Read the model definition and answer for the solid it produces. Units are mm, in the model's axes. A direction names the side the tool comes from. Coordinates: 2 decimals unless noted, no trailing zeros. Loops run counter-clockwise (first coordinate to the right, second up) from the corner with the lowest first, then second, coordinate; pieces in that order, holes last. Notation, with made-up numbers: (11, 5.25) - (30, 5.25) arc R25 cw to (30, 17.25) - close; hole circle Ø3 at (52, -24). An arc over 180 degrees is marked (long way). Use one line per item in the form item = value.
from build123d import *

# Parameters (mm, degrees)
SKETCH1_W           = 38.1
SKETCH1_H           = 12.7
BOSS_EXTRUDE1_DEPTH = 95.25
SKETCH2_R           = 54.61
SKETCH2_R_2         = 48.26
BOSS_EXTRUDE2_DEPTH = 6.35


with BuildPart() as part:
    # Sketch1 → Boss-Extrude1 (new body)
    with BuildSketch(Plane.XY):
        with Locations((0, -6.35)):
            Rectangle(SKETCH1_W, SKETCH1_H)
    extrude(amount=BOSS_EXTRUDE1_DEPTH)

    # Sketch2 → Boss-Extrude2 (add)
    with BuildSketch(Plane(origin=(0, 0, 0), x_dir=(-1, 0, 0), z_dir=(0, 0, -1))):
        with Locations((0, 49.53)):
            Circle(SKETCH2_R)
        with Locations((0, 49.53)):
            Circle(SKETCH2_R_2, mode=Mode.SUBTRACT)
    extrude(amount=-BOSS_EXTRUDE2_DEPTH)


solid = part.part
Item 1: The part is cut by section C-C on x = 0. Give the vertices of the cut face in (y, z), plus the area to 3 significant figures.
Results below:
outline = (-12.7, 0) - (1.27, 0) - (1.27, 6.35) - (0, 6.35) - (0, 95.25) - (-12.7, 95.25) - close; (97.79, 0) - (104.14, 0) - (104.14, 6.35) - (97.79, 6.35) - close
area = 1,260 mm²
Item 2: Each of these flat-tipped pins is pushed along its axis until it touches: P1, Ø6.5, axis at y = -4, z = 60, coming from the +X side; P2, Ø4, axis at y = -6.5, z = 35.5, coming from the -X side; P3, Ø5, axis at x = -40.5, y = 81, coming from the +Z side; P4, Ø2, axis at x = -8.5, y = 1.5, coming from the -Z side. Where does it stop, or does it pass through?
Results below:
P1 = 19.05
P2 = -19.05
P3 = 6.35
P4 = 0
Item 3: Which of the six approach directions +Z, -Z, +X, -X, +Y, -Y give full straight-line access (tool end or side, diameter ignored) to faces 1 (the flat face through (0, 0, 50)), 2 (the cylindrical face through (-22.269, 6.715, 3.131))?
Results below:
face_1 = +Z, +X, -X, +Y
face_2 = +Z, -Z
Item 4: The part is cut by section A-A on y = 49.53. Give the vertices of the cut face in (x, z).
Results below:
outline = (-54.61, 0) - (-48.26, 0) - (-48.26, 6.35) - (-54.61, 6.35) - close; (48.26, 0) - (54.61, 0) - (54.61, 6.35) - (48.26, 6.35) - close
Item 5: The part is cut by section D-D on z = 55.5. Give the vertices of the cut face in (x, y).
Results below:
outline = (-19.05, -12.7) - (19.05, -12.7) - (19.05, 0) - (-19.05, 0) - close
Item 6: The part is cut by section B-B on x = 45. Give the vertices of the cut face in (y, z).
Results below:
outline = (18.59, 0) - (32.09, 0) - (32.09, 6.35) - (18.59, 6.35) - close; (66.97, 0) - (80.47, 0) - (80.47, 6.35) - (66.97, 6.35) - close
Item 7: Find the intervals of material crossed by L1, parallel to X at y = 49, z = 4; L2, parallel to Y at x = 0, z = 3; L3, parallel to Y at x = 41, z = 5, in increasing order.
Results below:
L1 = -54.61 to -48.26, 48.26 to 54.61
L2 = -12.7 to 1.27, 97.79 to 104.14
L3 = 13.46 to 24.07, 74.99 to 85.6
